```python
from build123d import *

# Parameters (mm, degrees)
SKETCH_1_W           = 40
SKETCH_1_H           = 30
EXTRUDE_1_DEPTH      = 30
SKETCH_46_W          = 20
SKETCH_46_H          = 10
CUT_EXTRUDE_32_DEPTH = 59.309518948
CUT_EXTRUDE_33_DEPTH = 59.309518948
CUT_EXTRUDE_34_DEPTH = 20
EXTRUDE_2_DEPTH      = 10
CUT_EXTRUDE_35_DEPTH = 20
SKETCH_54_W          = 10
SKETCH_54_H          = 5
EXTRUDE_3_DEPTH      = 10


with BuildPart() as part:
    # 草圖1 → 填料-伸1 (new body)
    with BuildSketch(Plane.XY):
        with Locations((20, 15)):
            Rectangle(SKETCH_1_W, SKETCH_1_H)
    extrude(amount=-EXTRUDE_1_DEPTH)

    # 草圖46 → 除料-伸長32 (cut, through all)
    with BuildSketch(Plane.XY):
        Polygon((40, 30), (10, 30), (10, 20), (20, 20), (40, 20), align=None)
        with Locations((30, 15)):
            Rectangle(SKETCH_46_W, SKETCH_46_H)
    extrude(amount=-CUT_EXTRUDE_32_DEPTH, mode=Mode.SUBTRACT)

    # 草圖47 → 除料-伸長33 (cut, through all)
    with BuildSketch(Plane(origin=(0, 30, 0), x_dir=(1, 0, 0), z_dir=(0, 1, 0))):
        Polygon((20, 0), (20, 10), (30, 10), (30, 20), (40, 20), (40, 0), align=None)
    extrude(amount=-CUT_EXTRUDE_33_DEPTH, mode=Mode.SUBTRACT)

    # 草圖48 → 除料-伸長34 (cut)
    with BuildSketch(Plane.XY):
        Polygon((0, 30), (10, 20), (10, 30), align=None)
    extrude(amount=-CUT_EXTRUDE_34_DEPTH, mode=Mode.SUBTRACT)

    # 填料-伸長2: read off the stored shape, not the designer's step
    # 填料-伸長2 outline → 填料-伸長2 (add)
    with BuildSketch(Plane.YZ):
        Polygon((20, -30), (30, -30), (30, -20), (20, 0), align=None)
    extrude(amount=EXTRUDE_2_DEPTH)

    # 草圖52 → 除料-伸長35 (cut)
    with BuildSketch(Plane(origin=(40, 0, 0), x_dir=(0, 0, -1), z_dir=(1, 0, 0))):
        Polygon((20, 10), (20, 5), (30, 10), align=None)
        Polygon((10, 10), (10, 0), (20, 5), (20, 10), align=None)
    extrude(amount=-CUT_EXTRUDE_35_DEPTH, mode=Mode.SUBTRACT)

    # 草圖54 → 填料-伸長3 (add)
    with BuildSketch(Plane(origin=(20, 0, 0), x_dir=(0, 0, -1), z_dir=(1, 0, 0))):
        with Locations((25, 7.5)):
            Rectangle(SKETCH_54_W, SKETCH_54_H)
    extrude(amount=EXTRUDE_3_DEPTH)


solid = part.part
```
CAD build for the part. Positions are in the model's coordinates, mm. A direction names the side the tool comes from. Coordinates: 2 decimals unless noted, no trailing zeros. Loops run counter-clockwise (first coordinate to the right, second up) from the corner with the lowest first, then second, coordinate; pieces in that order, holes last. Notation, with made-up numbers: (11, -15.75) - (23, -15.75) arc R19 cw to (23, 7.25) - close; hole circle Ø2 at (51, 25). An arc over 180 degrees is marked (long way). Use CSV: the item, a comma, the result in double quotes. Start each with the question number.
Q1. Cut at B-B, the plane y = 20.5. List the corners of the cut face in (x, z).
Q2. 3-axis set-ups, long thin cutter, end or side, ignore diameter. For faces 1 (the flat face through (30, 1, -17)), 2 (the flat face through (5, 30, -25)), 3 (the flat face through (30, 8, -24)), 4 (the flat face through (25, 10, -25)): which of +Z, -Z, +X, -X, +Y, -Y reach the whole face in a straight line?
Q3. Probe probe 1 along X at (y, z) = (7.5, -16); probe 2 along X at (y, z) = (25.5, -22.5). List the from-to ranges inside material, lowest first. Write a range as from..to.
Q4. Drop flat-ended pins along their axis: P1, Ø11, axis at y = 24, z = -14, coming from the +X side; P2, Ø4, axis at x = 19.5, z = -20, coming from the +Y side; P3, Ø1, axis at x = 25, z = -25.5, coming from the +Y side. Give the stop position or say it passes through.
Q5. Cut at D-D, the plane z = -15. List the corners of the cut face in (x, y).
Q6. Cut at A-A, the plane z = -8.5. List the corners of the cut face in (x, y).
Q7. Cut at C-C, the plane x = 21. List the corners of the cut face in (y, z), then the cut area to 3 significant figures.
Here are the results:
1,outline,"(0, -30) - (10, -30) - (10, -1) - (9.5, -1) - (9.5, 0) - (0, 0) - close"
2,face 1,"+Z, +X, +Y, -Y"
2,face 2,"+Z, -Z, +X, -X, +Y"
2,face 3,"+Z, +X, +Y"
2,face 4,"+Z, -Z, +X, +Y"
3,probe 1,"0..20"
3,probe 2,"0..10"
4,P1,"x = 20"
4,P2,"y = 20"
4,P3,"y = 10"
5,outline,"(0, 0) - (30, 0) - (30, 2.5) - (20, 2.5) - (20, 20) - (10, 20) - (10, 27.5) - (2.5, 27.5) - (0, 30) - close"
6,outline,"(0, 0) - (20, 0) - (20, 20) - (10, 20) - (10, 24.25) - (5.75, 24.25) - (0, 30) - close"
7,outline,"(0, -30) - (10, -30) - (10, -20) - (5, -20) - (0, -10) - close"
7,area,"125 mm2"
